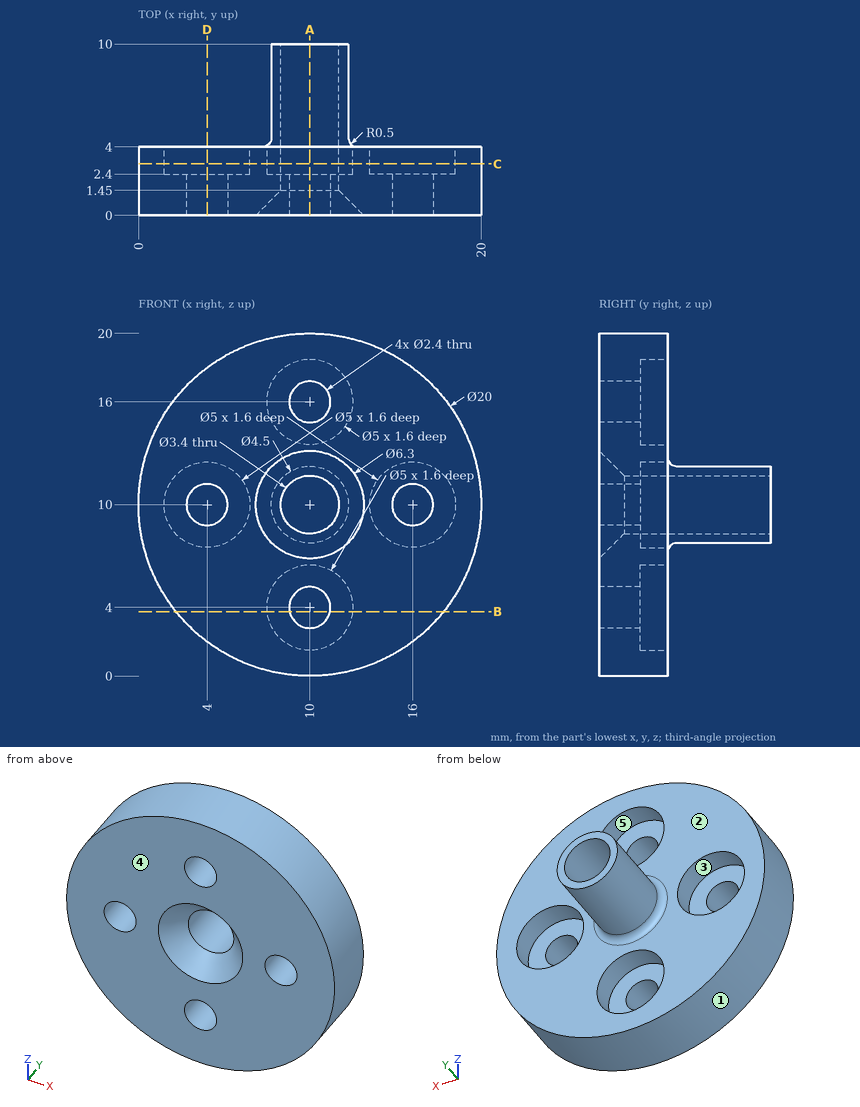
Here's the drawing with two shaded views (mm, measured from the low corner). I have some questions. A direction names the side the tool comes from. Give positions to 0.01 mm unless a question says otherwise; leave off trailing zeros. Order: outer loops, then holes, each group sorted by start corner. A loop starts at its lowest first (then second) coordinate and runs counter-clockwise, first axis right, second up.
Q1. If I drill on line 1 along X through (y, z) = (5.25, 10); line 2 along X through (y, z) = (3.75, 10.5); line 3 along Y through (x, z) = (5, 8.75), over which ranges is the centre line in solid material (lowest first)?
Q2. We'd pull the mould along X, two halves only. Please class the marked faces 1, 2 and 3: +X half, -X half, draft (parallel to the pull), parting line (faces both ways), or undercut.
Q3. Suppose I cut it at C-C, the plane y = 3. Write out the boundary of the cut face in (x, z), and give its area (3 significant figures).
Q4. Suppose I cut it at B-B, the plane z = 3.75. Write out the boundary of the cut face in (x, y).
Q5. Suppose I cut it at A-A, the plane x = 10. Count the separate pieces of the cut face and the enclosed holes in it, and give its area (3 significant figures).
Q6. For the marked faces 4 and 5, which set-ups out of +Z, -Z, +X, -X, +Y, -Y let a thin tool reach every point of the face, with its end or its side?
Q7. I'm going to push flat-ended pins straight in: P1, Ø3, axis at x = 2.5, z = 9, coming from the +Y side; P2, Ø3, axis at x = 10, z = 16, coming from the +Y side; P3, Ø1.5, axis at x = 11.5, y = 5, coming from the +Z side. Where does each tip first touch, or does it pass through?
Q8. Suppose I cut it at D-D, the plane x = 4. Write out the boundary of the cut face in (y, z), and give its area (3 significant figures).
Solution:
1. line 1: x = 7.75 to 8.3, 11.7 to 12.25
1. line 2: x = 0.01 to 1.55, 6.45 to 8.38, 11.62 to 13.55, 18.45 to 19.99
1. line 3: y = 0 to 2.4
2. face 1: parting line
2. face 2: draft
2. face 3: undercut
3. outline: circle Ø20 at (10, 10); hole circle Ø5 at (4, 10); hole circle Ø5 at (10, 4); hole circle Ø5 at (10, 16); hole circle Ø3.4 at (10, 10); hole circle Ø5 at (16, 10)
3. area: 227 mm2
4. outline: (2.19, 0) - (8.83, 0) - (8.83, 2.4) - (7.51, 2.4) - (7.51, 4) - (2.19, 4) - close; (11.17, 0) - (17.81, 0) - (17.81, 4) - (12.49, 4) - (12.49, 2.4) - (11.17, 2.4) - close
5. separate pieces: 4
5. enclosed holes: 0
5. area: 43.5 mm2
6. face 4: +Z, -Z, +X, -X, -Y
6. face 5: +Y
7. P1: stops at y = 4
7. P2: stops at y = 2.4
7. P3: stops at z = 12.12
8. outline: (0, 2) - (4, 2) - (4, 7.5) - (2.4, 7.5) - (2.4, 8.8) - (0, 8.8) - close; (0, 11.2) - (2.4, 11.2) - (2.4, 12.5) - (4, 12.5) - (4, 18) - (0, 18) - close
8. area: 50.2 mm2
